```python
from build123d import *

# Parameters (mm, degrees)
F0_R     = 1.017764
F0_R_2   = 1
F1_DEPTH = 2
F2_R     = 1
F3_DEPTH = 5.2
F4_R     = 1.5
F4_R_2   = 1
F5_DEPTH = 3.5
F6_R     = 1
F7_DEPTH = 10


with BuildPart() as f1:
    # F0 (on Front) → F1 (new body)
    with BuildSketch(Plane.XZ):
        Polygon((-11.371579, 18), (-15, 18), (-15, -18), (15, -18), (15, 18), (5.371579, 18), align=None)
        with Locations((-9, -15)):
            Circle(F0_R, mode=Mode.SUBTRACT)
        with Locations((-0.812178, -12.593267)):
            Circle(F0_R_2, mode=Mode.SUBTRACT)
        with Locations((9, -15)):
            Circle(F0_R, mode=Mode.SUBTRACT)
        with Locations((11.312178, -5.593267)):
            Circle(F0_R_2, mode=Mode.SUBTRACT)
        with Locations((-11.312178, 5.593267)):
            Circle(F0_R_2, mode=Mode.SUBTRACT)
        with Locations((-9, 15)):
            Circle(F0_R_2, mode=Mode.SUBTRACT)
        with Locations((0.812178, 12.593267)):
            Circle(F0_R_2, mode=Mode.SUBTRACT)
        with Locations((9, 15)):
            Circle(F0_R_2, mode=Mode.SUBTRACT)
    extrude(amount=F1_DEPTH)

    # F2 (on face) → F3 (join)
    with BuildSketch(Plane.XZ.offset(2)):
        with Locations((-11.312178, 5.593267)):
            Circle(F2_R)
        with Locations((-0.812178, -12.593267)):
            Circle(F2_R)
        with Locations((0.812178, 12.593267)):
            Circle(F2_R)
        with Locations((11.312178, -5.593267)):
            Circle(F2_R)
        Polygon((14.727241, -6.50833), (1.727241, 16.00833), (-14.727241, 6.50833), (-1.727241, -16.00833), align=None)
        with Locations((-0.812178, -12.593267)):
            Circle(F2_R, mode=Mode.SUBTRACT)
        with Locations((11.312178, -5.593267)):
            Circle(F2_R, mode=Mode.SUBTRACT)
        with Locations((-11.312178, 5.593267)):
            Circle(F2_R, mode=Mode.SUBTRACT)
        with Locations((0.812178, 12.593267)):
            Circle(F2_R, mode=Mode.SUBTRACT)
    extrude(amount=F3_DEPTH)

    # F4 (on face) → F5 (cut)
    with BuildSketch(Plane(origin=(0, 0, 0), x_dir=(-1, 0, 0), z_dir=(0, 1, 0))):
        with Locations((-11.312178, -5.593267)):
            Circle(F4_R)
        with Locations((-11.312178, -5.593267)):
            Circle(F4_R_2, mode=Mode.SUBTRACT)
        with Locations((0.812178, -12.593267)):
            Circle(F4_R)
        with Locations((0.812178, -12.593267)):
            Circle(F4_R_2, mode=Mode.SUBTRACT)
        with Locations((-0.812178, 12.593267)):
            Circle(F4_R)
        with Locations((-0.812178, 12.593267)):
            Circle(F4_R_2, mode=Mode.SUBTRACT)
        with Locations((11.312178, 5.593267)):
            Circle(F4_R)
        with Locations((11.312178, 5.593267)):
            Circle(F4_R_2, mode=Mode.SUBTRACT)
    extrude(amount=-F5_DEPTH, mode=Mode.SUBTRACT)

    # F6 (on face) → F7 (cut)
    with BuildSketch(Plane(origin=(0, 0, 0), x_dir=(-1, 0, 0), z_dir=(0, 1, 0))):
        with Locations((-0.812178, 12.593267)):
            Circle(F6_R)
        with Locations((11.312178, 5.593267)):
            Circle(F6_R)
        with Locations((0.812178, -12.593267)):
            Circle(F6_R)
        with Locations((-11.312178, -5.593267)):
            Circle(F6_R)
    extrude(amount=-F7_DEPTH, mode=Mode.SUBTRACT)


solid = f1.part
```
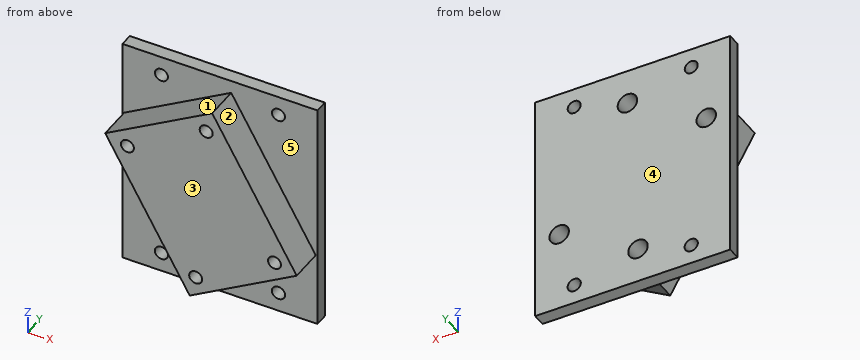
The model under review builds one solid part; all positions refer to its coordinate system, in mm. Face numbers are marked on the shaded views. A direction names the side the tool comes from. Round coordinates to 2 decimals unless told otherwise and drop trailing zeros. Write each loop counter-clockwise with the first axis right and the second up, starting at its lowest first coordinate (ties: lowest second). Pieces come first, ordered by that corner, then holes.
(1) Wall thickness on L1, parallel to Z at x = -9, y = -0.65; L2, parallel to Z at x = 12, y = -5.25; L3, parallel to Y at x = -13.5, z = 10: over which ranges is each line inside the solid? List them lowest first.
(2) We need section B-B on z = 15. Give the boundary of the cut face in (x, y), and give its area (3 significant figures).
(3) Machinability: for the marked faces 4 and 5, which of the approach directions +Z, -Z, +X, -X, +Y, -Y give a long, thin tool a straight path to every point of the face, cutting with its end or side? Answer none if there is none.
(4) We need section A-A on x = 9. Give the boundary of the cut face in (y, z).
(5) We need section C-C on x = -11.75. Give the boundary of the cut face in (y, z), and give its area (3 significant figures).
(6) Insertion check: pin 1 (2.5 mm diameter, centred on x = -9, z = 15, fed in from +Y); pin 2 (4 mm diameter, centred on y = -6, z = -14, fed in from -X); pin 3 (2.5 mm diameter, centred on x = 9, z = 15, fed in from -Y); pin 4 (1.5 mm diameter, centred on x = -5, y = -5, fed in from -Z). Each pin has a flat end and moves straight along its axis. Give the tip position at first contact, or say it passes through.
(7) We need section D-D on y = -5. Give the boundary of the cut face in (x, z).
(8) Mouldability with a two-part tool opening along X and no side actions: class the marked faces 1, 2 and 3 as +X half, -X half, draft (parallel to the pull), parting line (faces both ways), or undercut.
Findings below:
1. L1: z = -18 to -16.02, -13.98 to 14, 16 to 18
1. L2: z = -8.08 to -6.32, -4.87 to -1.78
1. L3: y = -2 to 0
2. outline: (-15, -2) - (-10, -2) - (-10, 0) - (-15, 0) - close; (-8, -2) - (-0.02, -2) - (-0.02, -7.2) - (2.31, -7.2) - (2.31, -2) - (8, -2) - (8, 0) - (-8, 0) - close; (10, -2) - (15, -2) - (15, 0) - (10, 0) - close
2. area: 64.1 mm2
3. face 4: +Z, -Z, +X, -X, +Y
3. face 5: -Y
4. outline: (-7.2, -9.81) - (-2, -9.81) - (-2, -13.98) - (0, -13.98) - (0, 14) - (-2, 14) - (-2, 3.41) - (-7.2, 3.41) - close; (-2, -18) - (0, -18) - (0, -16.02) - (-2, -16.02) - close; (-2, 16) - (0, 16) - (0, 18) - (-2, 18) - close
5. outline: (-7.2, 1.35) - (-2, 1.35) - (-2, -18) - (0, -18) - (0, 4.16) - (-3.5, 4.16) - (-3.5, 4.69) - (-7.2, 4.69) - close; (-7.2, 6.49) - (-3.5, 6.49) - (-3.5, 7.03) - (0, 7.03) - (0, 18) - (-2, 18) - (-2, 8.23) - (-7.2, 8.23) - close
5. area: 91.1 mm2
6. pin 1: stops at y = 0
6. pin 2: stops at x = -4.04
6. pin 3: stops at y = -2
6. pin 4: stops at z = -11.64
7. outline: (-14.73, 6.51) - (-1.73, -16.01) - (14.73, -6.51) - (1.73, 16.01) - close; hole circle Ø2 at (-11.31, 5.59); hole circle Ø2 at (-0.81, -12.59); hole circle Ø2 at (0.81, 12.59); hole circle Ø2 at (11.31, -5.59)
8. face 1: -X half
8. face 2: +X half
8. face 3: draft
